Here's how the part is built. I have some questions about the finished solid (model axes, mm). A direction names the side the tool comes from. Give positions to 0.01 mm unless a question says otherwise; leave off trailing zeros. Loops run counter-clockwise (first coordinate to the right, second up) from the corner with the lowest first, then second, coordinate; pieces in that order, holes last. Notation, with made-up numbers: (84.5, -33) - (116.5, -33) arc R7 ccw to (116.5, -29) - close; hole circle Ø7 at (-22, -15). An arc over 180 degrees is marked (long way). Return JSON: item names as keys, results as strings. Group by question number.
(1) If we section it at C-C (y = 6.25): Please give me the cut outline in (x, z).
(2) On a 3-axis mill with a long thin cutter (end or side, diameter ignored), from which of +Z, -Z, +X, -X, +Y, -Y can I reach the whole of each face in a straight line? I mean faces 1 (the cylindrical face through (-46.05, 3.72, -6.32)), 2 (the flat face through (-19.99, 1, 38)), 3 (the flat face through (-29, 0, 38)). Say none if no direction works.
(3) If we section it at B-B (x = 22.5): Please give me the cut outline in (y, z).
(4) For P1, Ø1, axis at y = 1, z = 38, coming from the +X side; P2, Ø6, axis at x = -8, z = 31, coming from the -Y side; P3, Ø1.6, axis at x = -31, z = -11.5, coming from the +Y side, each with a flat end and sliding along its axis, tell me the tip position at first contact or that it passes through.
(5) If we section it at D-D (x = -30): Please give me the cut outline in (y, z).
(6) If we mould it in two halves opening along Y, with no side actions, what happens to faces 4 (the cylindrical face through (35.944, 2.585, 0.265)), 5 (the flat face through (-7, 5, -10.364)), 6 (the flat face through (-16, 2.377, 38))? For each: released by +Y, released by -Y, zero draft, split by the parting line, or undercut.
(7) I need wall thicknesses on probe 1 along Z at (x, y) = (-39.5, 3.75); probe 2 along Z at (x, y) = (-26, 2); probe 3 along Z at (x, y) = (21, 10.25). Which ranges of each line are inside material? Lowest first, please. Write a range as [from, to].
(8) If we section it at A-A (x = -14): Please give me the cut outline in (y, z).
```python
from build123d import *

# Parameters (mm, degrees)
F1_DEPTH    = 12.7
F2_T        = -2.54
F3_R        = 2.5336521523
F4_DEPTH    = 25.4
F5_W        = 12.6487519592
F5_H        = 3.011607565
F6_DEPTH    = 2.032
F7_T1_DEPTH = 51.1041796342
F7_T3_DEPTH = 73.1048124282
F7_T5_DEPTH = 50.4994199847
F7_T7_DEPTH = 50.8
F8_W        = 7.2596892715
F8_H        = 2.5458435994
F8_W_2      = 8.1038391218
F8_H_2      = 2.3770136759
F9_DEPTH    = 2.032
F11_DEPTH   = 5.334
F12_DEPTH   = 10.16
F13_R       = 5.08
F14_R       = 2.6429379381
F15_DEPTH   = 25.4


# Not quite as in the source:
# - a fillet or chamfer that OpenCascade refuses, or shapes differently, is made with other operations: its cross-section is extruded or revolved along the edge and cut away or added


with BuildPart() as f1:
    # F0 (on Front) → F1 (new body, symmetric)
    with BuildSketch(Plane.XZ):
        Polygon((37.1957607567, 37.33773157), (-50.5407974124, 37.33773157), (-49.9729253352, -10.3637007996), (37.1957607567, -10.3637007996), align=None)
    extrude(amount=F1_DEPTH, both=True)

    # F2
    f2_openings = [f1.faces().sort_by_distance(p)[0] for p in [
        (-6.530704, -12.7, 13.512828),
    ]]
    offset(amount=F2_T, openings=f2_openings)

    # F3 (on face) → F4 (cut)
    with BuildSketch(Plane.XZ.offset(-10.16)):
        with Locations((-44.7698123753, 30.0145167857)):
            Circle(F3_R)
    extrude(amount=-F4_DEPTH, mode=Mode.SUBTRACT)

    # F5 (on face) → F6 (join)
    with BuildSketch(Plane(origin=(0, 0, -10.3637007996), x_dir=(1, 0, 0), z_dir=(0, 0, -1))):
        with Locations((-34.2319430783, -6.4247637056)):
            Rectangle(F5_W, F5_H)
    extrude(amount=F6_DEPTH)

    # F7: fillet of radius 5.08 on 5 edges, made by hand

    # F7_s2 → F7_t1 (cut)
    with BuildSketch(Plane.XZ.offset(-25.5520898171)):
        with BuildLine():
            ThreePointArc((-50.4796015492, 32.19725989), (-49.0133806513, 35.8283900433), (-45.3999614856, 37.33773157))
            Line((-45.3999614856, 37.33773157), (-50.5407974124, 37.33773157))
            Line((-50.5407974124, 37.33773157), (-50.4796015492, 32.19725989))
        make_face()
    extrude(amount=F7_T1_DEPTH, mode=Mode.SUBTRACT)

    # F7_s4 → F7_t3 (cut)
    with BuildSketch(Plane(origin=(-0.602773104, 0, 50.6331295472), x_dir=(0, 1, 0), z_dir=(0.011903874, 0, -0.9999291464))):
        with BuildLine():
            ThreePointArc((12.7, -45.0127527613), (11.2121024484, -48.6048552097), (7.62, -50.0927527613))
            Line((7.62, -50.0927527613), (12.7, -50.0927527613))
            Line((12.7, -50.0927527613), (12.7, -45.0127527613))
        make_face()
    extrude(amount=F7_T3_DEPTH, mode=Mode.SUBTRACT)

    # F7_s6 → F7_t5 (cut)
    with BuildSketch(Plane.XZ.offset(-25.2497099923)):
        with BuildLine():
            ThreePointArc((-44.9530413382, -10.3637007996), (-48.5236998115, -8.8971199654), (-50.0326814019, -5.3441724797))
            Line((-50.0326814019, -5.3441724797), (-49.9729253352, -10.3637007996))
            Line((-49.9729253352, -10.3637007996), (-44.9530413382, -10.3637007996))
        make_face()
    extrude(amount=F7_T5_DEPTH, mode=Mode.SUBTRACT)

    # F7_s8 → F7_t7 (cut)
    with BuildSketch(Plane.XZ.offset(-25.4)):
        with BuildLine():
            ThreePointArc((32.1157607567, -10.3637007996), (35.7078632052, -8.8758032481), (37.1957607567, -5.2837007996))
            Line((37.1957607567, -5.2837007996), (37.1957607567, -10.3637007996))
            Line((37.1957607567, -10.3637007996), (32.1157607567, -10.3637007996))
        make_face()
        with BuildLine():
            ThreePointArc((37.1957607567, 32.25773157), (35.7078632052, 35.8498340184), (32.1157607567, 37.33773157))
            Line((32.1157607567, 37.33773157), (37.1957607567, 37.33773157))
            Line((37.1957607567, 37.33773157), (37.1957607567, 32.25773157))
        make_face()
    extrude(amount=F7_T7_DEPTH, mode=Mode.SUBTRACT)

    # F8 (on face) → F9 (join)
    with BuildSketch(Plane.XY.offset(37.33773157)):
        with Locations((-28.5155698657, 1.2729217997)):
            Rectangle(F8_W, F8_H)
        with Locations((-15.9377348609, 1.1885068379)):
            Rectangle(F8_W_2, F8_H_2)
    extrude(amount=F9_DEPTH)

    # F10 (on face) → F11 (cut)
    with BuildSketch(Plane.XZ.offset(-10.16)):
        with BuildLine():
            add(Edge.make_bspline(
                [(-44.4320701063, 24.525936693), (-48.8002594528, 24.525936693), (-46.6161647795, 18.5632575303), (-44.4320701063, 12.6005783677), (-42.247975433, 18.5632575303), (-40.0638807598, 24.525936693), (-44.4320701063, 24.525936693)],
                knots=[0, 0, 0, 2.0943951024, 2.0943951024, 4.1887902048, 4.1887902048, 6.2831853072, 6.2831853072, 6.2831853072], degree=2, weights=[1, 0.5, 1, 0.5, 1, 0.5, 1]))
        make_face()
    extrude(amount=-F11_DEPTH, mode=Mode.SUBTRACT)

    # F12 (cut): a face of the model
    f12_faces = [f1.faces().sort_by_distance(p)[0] for p in [
        (-48.3034140755, -12.7, 35.1268251117),
    ]]
    extrude(f12_faces, amount=-F12_DEPTH, mode=Mode.SUBTRACT)

    # F13
    f13_edges = [f1.edges().sort_by_distance(p)[0] for p in [
        (-47.462983, 3.81, -7.823701),
        (-47.970379, 3.81, 34.797732),
        (34.655761, 3.81, -7.823701),
        (34.655761, 3.81, 34.797732),
    ]]
    fillet(f13_edges, radius=F13_R)

    # F14 (on face) → F15 (cut)
    with BuildSketch(Plane.YZ.offset(37.1957607567)):
        with Locations((4.6823634766, 1.8731907476)):
            Circle(F14_R)
    extrude(amount=-F15_DEPTH, mode=Mode.SUBTRACT)


solid = f1.part
```
Values:
{
 "1": {"outline": "(-50.48, 32.2) - (-50.03, -5.34) arc R5.08 ccw to (-44.95, -10.36) - (-40.56, -10.36) - (-40.56, -12.4) - (-27.91, -12.4) - (-27.91, -10.36) - (32.12, -10.36) arc R5.08 ccw to (37.2, -5.28) - (37.2, -0.25) - (34.66, -0.25) - (34.66, -2.74) arc R5.08 cw to (29.58, -7.82) - (-42.44, -7.82) arc R5.08 cw to (-47.52, -2.8) - (-47.91, 29.66) arc R5.08 cw to (-42.83, 34.8) - (29.58, 34.8) arc R5.08 cw to (34.66, 29.72) - (34.66, 4) - (37.2, 4) - (37.2, 32.26) arc R5.08 ccw to (32.12, 37.34) - (-45.4, 37.34) arc R5.08 ccw to start"},
 "2": {"face 1": "-Y", "face 2": "+Z, +Y, -Y", "face 3": "+Z, +X, -X, -Y"},
 "3": {"outline": "(-2.54, -10.36) - (12.7, -10.36) - (12.7, 37.34) - (-2.54, 37.34) - (-2.54, 34.8) - (10.16, 34.8) - (10.16, -7.82) - (-2.54, -7.82) - close"},
 "4": {"P1": "x = -11.89", "P2": "y = 10.16", "P3": "y = 7.93"},
 "5": {"outline": "(-2.54, -10.36) - (4.92, -10.36) - (4.92, -12.4) - (7.93, -12.4) - (7.93, -10.36) - (12.7, -10.36) - (12.7, 37.34) - (2.55, 37.34) - (2.55, 39.37) - (0, 39.37) - (0, 37.34) - (-2.54, 37.34) - (-2.54, 34.8) - (10.16, 34.8) - (10.16, -7.82) - (-2.54, -7.82) - close"},
 "6": {"face 4": "undercut", "face 5": "zero draft", "face 6": "released by +Y"},
 "7": {"probe 1": "[-10.36, -7.82], [34.8, 37.34]", "probe 2": "[-10.36, -7.82], [34.8, 39.37]", "probe 3": "[-10.36, 37.34]"},
 "8": {"outline": "(-2.54, -10.36) - (12.7, -10.36) - (12.7, 37.34) - (2.38, 37.34) - (2.38, 39.37) - (0, 39.37) - (0, 37.34) - (-2.54, 37.34) - (-2.54, 34.8) - (10.16, 34.8) - (10.16, -7.82) - (-2.54, -7.82) - close"}
}
